Can you work these out from the model? Positions are in its coordinate system, mm. Face numbers are marked on the shaded views. Coordinates: 2 decimals unless noted, no trailing zeros. Loops run counter-clockwise (first coordinate to the right, second up) from the corner with the lowest first, then second, coordinate; pieces in that order, holes last. Notation, with made-up numbers: (4.25, -27.75) - (10.25, -27.75) arc R31 ccw to (10.25, -1.75) - close; hole circle Ø3 at (42, 48.25). An arc over 180 degrees is marked (long way). Put each result on its own line as item: value. Start each with the question number.
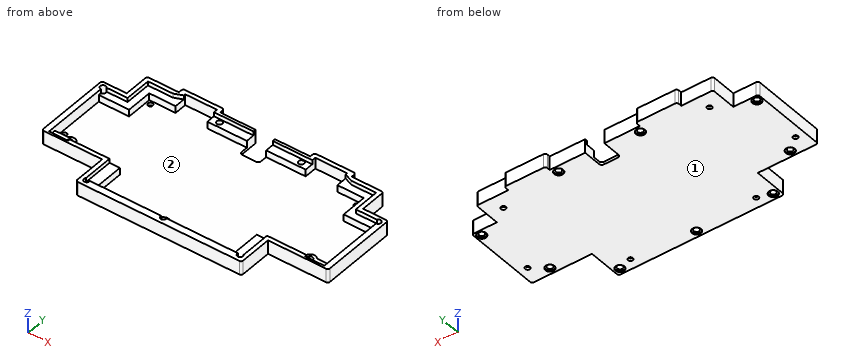
from build123d import *

# Parameters (mm, degrees)
PAD002_DEPTH    = 10
POCKET006_DEPTH = 8
POCKET007_DEPTH = 3
PAD003_START    = -3
SKETCH017_R     = 4
PAD003_DEPTH    = 7
SKETCH016_R     = 2
POCKET008_DEPTH = 10.001
POCKET009_START = -9
SKETCH018_R     = 3.25
POCKET009_DEPTH = 5
POCKET010_DEPTH = 10.001
SKETCH020_R     = 1.75
POCKET011_DEPTH = 10.001
FILLET001_R     = 1.5


with BuildPart() as part:
    # Sketch013 → Pad002 (new body)
    with BuildSketch(Plane.XY):
        Polygon((-103.725, 5.8125), (-103.725, 61.8625), (-85.675, 61.8625), (-85.675, 80.9125), (-62.625, 80.9125), (-62.625, 84.7225), (-32.625, 84.7225), (-32.625, 80.9125), (32.625, 80.9125), (32.625, 84.7225), (62.625, 84.7225), (62.625, 80.9125), (85.675, 80.9125), (85.675, 61.8625), (103.725, 61.8625), (103.725, 5.8125), (60.075, 5.8125), (60.075, -19), (-60.075, -19), (-60.075, 5.8125), align=None)
    extrude(amount=-PAD002_DEPTH)

    # Sketch014 → Pocket006 (cut)
    with BuildSketch(Plane.XY):
        Polygon((-99.725, 12.8125), (-85.725, 12.8125), (-85.725, 8.8125), (-49.575, 8.8125), (-49.575, -14), (49.575, -14), (49.575, 8.8125), (85.725, 8.8125), (85.725, 12.8125), (99.725, 12.8125), (99.725, 53.8625), (77.725, 53.8625), (77.725, 72.7225), (58.625, 72.7225), (58.625, 81.7225), (35.625, 81.7225), (35.625, 72.7225), (-35.625, 72.7225), (-35.625, 81.7225), (-58.625, 81.7225), (-58.625, 72.7225), (-77.725, 72.7225), (-77.725, 53.8625), (-99.725, 53.8625), align=None)
    extrude(amount=-POCKET006_DEPTH, mode=Mode.SUBTRACT)

    # Sketch015 → Pocket007 (cut)
    with BuildSketch(Plane.XY):
        Polygon((-57.075, -14), (-57.075, 8.8125), (-85.725, 8.8125), (-85.725, 7.3125), (-99.725, 7.3125), (-99.725, 58.8625), (-82.675, 58.8625), (-82.675, 77.9125), (-64.625, 77.9125), (-55.481, 81.7225), (-35.625, 81.7225), (-35.625, 78.9125), (35.625, 78.9125), (35.625, 81.7225), (55.481, 81.7225), (64.625, 77.9125), (82.675, 77.9125), (82.675, 58.8625), (99.725, 58.8625), (99.725, 7.3125), (85.725, 7.3125), (85.725, 8.8125), (57.075, 8.8125), (57.075, -14), align=None)
    extrude(amount=-POCKET007_DEPTH, mode=Mode.SUBTRACT)

    # Sketch017 → Pad003 (join)
    with BuildSketch(Plane.XY.offset(PAD003_START)):
        with Locations((-87.075, 10.3125)):
            Circle(SKETCH017_R)
        with Locations((87.075, 10.3125)):
            Circle(SKETCH017_R)
        with Locations((0, -14.5)):
            Circle(SKETCH017_R)
    extrude(amount=-PAD003_DEPTH)

    # Sketch016 → Pocket008 (cut, through all)
    with BuildSketch(Plane.XY):
        with Locations((-29.625, 76.4125)):
            Circle(SKETCH016_R)
        with Locations((29.625, 76.4125)):
            Circle(SKETCH016_R)
        with Locations((87.075, 10.3125)):
            Circle(SKETCH016_R)
        with Locations((55.575, -14.5)):
            Circle(SKETCH016_R)
        with Locations((-55.575, -14.5)):
            Circle(SKETCH016_R)
        with Locations((-87.075, 10.3125)):
            Circle(SKETCH016_R)
        with Locations((99.725, 57.8625)):
            Circle(SKETCH016_R)
        with Locations((-99.725, 57.8625)):
            Circle(SKETCH016_R)
        with Locations((0, -14.5)):
            Circle(SKETCH016_R)
    extrude(amount=-POCKET008_DEPTH, mode=Mode.SUBTRACT)

    # Sketch018 → Pocket009 (cut)
    with BuildSketch(Plane.XY.offset(POCKET009_START)):
        with Locations((-99.725, 57.8625)):
            Circle(SKETCH018_R)
        with Locations((-87.075, 10.3125)):
            Circle(SKETCH018_R)
        with Locations((-55.575, -14.5)):
            Circle(SKETCH018_R)
        with Locations((55.575, -14.5)):
            Circle(SKETCH018_R)
        with Locations((87.075, 10.3125)):
            Circle(SKETCH018_R)
        with Locations((99.725, 57.8625)):
            Circle(SKETCH018_R)
        with Locations((29.625, 76.4125)):
            Circle(SKETCH018_R)
        with Locations((-29.625, 76.4125)):
            Circle(SKETCH018_R)
        with Locations((0, -14.5)):
            Circle(SKETCH018_R)
    extrude(amount=-POCKET009_DEPTH, mode=Mode.SUBTRACT)

    # Sketch019 (on Face5 of Pocket009) → Pocket010 (cut, through all)
    with BuildSketch(Plane(origin=(0, 0, -10), x_dir=(1, 0, 0), z_dir=(0, 0, -1))):
        with BuildLine():
            Line((0, -80.9125), (7, -80.9125))
            Line((7, -80.9125), (7, -67.9125))
            ThreePointArc((7, -67.9125), (6.414214, -66.498286), (5, -65.9125))
            Line((5, -65.9125), (0, -65.9125))
            Line((-5, -65.9125), (0, -65.9125))
            ThreePointArc((-5, -65.9125), (-6.414214, -66.498286), (-7, -67.9125))
            Line((-7, -80.9125), (-7, -67.9125))
            Line((0, -80.9125), (-7, -80.9125))
        make_face()
    extrude(amount=-POCKET010_DEPTH, mode=Mode.SUBTRACT)

    # Sketch020 → Pocket011 (cut, through all)
    with BuildSketch(Plane.XY):
        with Locations((-97.075, 18.3125)):
            Circle(SKETCH020_R)
        with Locations((-74.725, 69.8625)):
            Circle(SKETCH020_R)
        with Locations((74.725, 69.8625)):
            Circle(SKETCH020_R)
        with Locations((97.075, 18.3125)):
            Circle(SKETCH020_R)
        with Locations((-45.575, -11.5)):
            Circle(SKETCH020_R)
        with Locations((45.575, -11.5)):
            Circle(SKETCH020_R)
    extrude(amount=-POCKET011_DEPTH, mode=Mode.SUBTRACT)

    # Fillet001
    fillet001_edges = [part.edges().sort_by_distance(p)[0] for p in [
        (-60.075, -19, -5),
        (-103.725, 5.8125, -5),
        (-103.725, 61.8625, -5),
        (-85.675, 80.9125, -5),
        (-62.625, 84.7225, -5),
        (-32.625, 84.7225, -5),
        (32.625, 84.7225, -5),
        (62.625, 84.7225, -5),
        (85.675, 80.9125, -5),
        (103.725, 61.8625, -5),
        (103.725, 5.8125, -5),
        (60.075, -19, -5),
    ]]
    fillet(fillet001_edges, radius=FILLET001_R)


solid = part.part
Q1. We'd pull the mould along X, two halves only. Please class the marked faces 1 and 2: released by +X, released by -X, zero draft, split by the parting line, or undercut.
Q2. I want a section at C-C on x = 37.5. List the corners of the cut face in (y, z) for me, and give its area (3 significant figures).
Q3. Will these pins go through, and if not, where does the flat tip stop? pin 1 (1.9 mm diameter, centred on x = -18.5, y = 74.5, fed in from +Z); pin 2 (2.5 mm diameter, centred on y = 66.5, z = -1, fed in from +X) (3 decimals); pin 3 (5.5 mm diameter, centred on x = -74.72, y = 69.86, fed in from +Z); pin 4 (3.5 mm diameter, centred on x = -99.72, y = 57.86, fed in from +Z).
Q4. I want a section at A-A on x = 0. List the corners of the cut face in (y, z) for me.
Q5. I want a section at B-B on y = -7.5. List the corners of the cut face in (x, z) for me (3 decimals), and give its area (3 significant figures).
Q6. Please list where these lines run through material, in increasing order: line 1 along Y through (x, z) = (-87, -5); line 2 along X through (y, z) = (10, -5.5) (3 decimals); line 3 along X through (y, z) = (-14.5, -3.25) (3 decimals). Write a range as [from, to].
Q7. I want a section at D-D on z = -6.25. Count the separate pieces of the cut face and the enclosed holes in it, and give its area (3 significant figures).
Calculated:
1. face 1: zero draft
1. face 2: undercut
2. outline: (-19, -10) - (84.72, -10) - (84.72, 0) - (81.72, 0) - (81.72, -8) - (-14, -8) - (-14, 0) - (-19, 0) - close
2. area: 271 mm2
3. pin 1: z = -3
3. pin 2: x = 85.675
3. pin 3: z = -8
3. pin 4: through
4. outline: (-19, -10) - (-17.75, -10) - (-17.75, -9) - (-16.5, -9) - (-16.5, 0) - (-19, 0) - close; (-12.5, -9) - (-11.25, -9) - (-11.25, -10) - (65.91, -10) - (65.91, -8) - (-10.5, -8) - (-10.5, -3) - (-12.5, -3) - close
5. outline: (-60.075, -10) - (60.075, -10) - (60.075, 0) - (57.075, 0) - (57.075, -3) - (49.575, -3) - (49.575, -8) - (-49.575, -8) - (-49.575, -3) - (-57.075, -3) - (-57.075, 0) - (-60.075, 0) - close
5. area: 363 mm2
6. line 1: [5.81, 8.31], [12.31, 14.31], [53.86, 61.86]
6. line 2: [-103.725, -89.05], [-85.1, -83.087], [83.087, 85.1], [89.05, 103.725]
6. line 3: [-60.075, -57.575], [-53.575, -2], [2, 53.575], [57.575, 60.075]
7. separate pieces: 1
7. enclosed holes: 9
7. area: 3,440 mm2
